from build123d import *

# Parameters (mm, degrees)
BOSS_EXTRUDE1_DEPTH = 25.4
SKETCH2_W           = 3.81
SKETCH2_H           = 30.913886478
CUT_EXTRUDE1_DEPTH  = 24.638
SKETCH3_R           = 0.1905
BOSS_EXTRUDE2_DEPTH = 27.94


with BuildPart() as part:
    # Sketch1 → Boss-Extrude1 (new body)
    with BuildSketch(Plane(origin=(0, 0, 0), x_dir=(0, 1, 0), z_dir=(0, 0, 1))):
        with BuildLine():
            Line((38.1, 31.396083107), (38.1, 54.3969813))
            Line((38.1, 54.3969813), (-38.1, 54.3969813))
            Line((-38.1, 54.3969813), (-38.1, 29.686927473))
            ThreePointArc((-38.1, 29.686927473), (-47.228063928, 16.31611269), (-50.79728762, 0.524948031))
            ThreePointArc((-50.79728762, 0.524948031), (-0.262477519, -50.799321901), (50.8, 0))
            ThreePointArc((50.8, 0), (47.722223419, 17.021685566), (38.1, 31.396083107))
        make_face()
        with BuildLine():
            Line((-38.1, 16.2969813), (-43.366277143, 9.755434728))
            ThreePointArc((-43.366277143, 9.755434728), (7.077931126, -43.882859877), (38.1, 22.895250599))
            ThreePointArc((38.1, 22.895250599), (-1.174082446, 33.154986969), (-38.1, 16.2969813))
        make_face(mode=Mode.SUBTRACT)
    extrude(amount=BOSS_EXTRUDE1_DEPTH)

    # Sketch2 → Cut-Extrude1 (cut)
    with BuildSketch(Plane.XY.offset(25.4)):
        with Locations((-52.2379813, 0.268816404)):
            Rectangle(SKETCH2_W, SKETCH2_H)
    extrude(amount=-CUT_EXTRUDE1_DEPTH, mode=Mode.SUBTRACT)

    # Sketch3 → Boss-Extrude2 (add)
    with BuildSketch(Plane.XY.offset(0.762)):
        with Locations((-52.2379813, -12.905010915)):
            Circle(SKETCH3_R)
        with Locations((-52.2379813, -9.095010915)):
            Circle(SKETCH3_R)
        with Locations((-52.2379813, -5.285010915)):
            Circle(SKETCH3_R)
        with Locations((-52.2379813, -1.475010915)):
            Circle(SKETCH3_R)
        with Locations((-52.2379813, 2.334989085)):
            Circle(SKETCH3_R)
        with Locations((-52.2379813, 6.144989085)):
            Circle(SKETCH3_R)
        with Locations((-52.2379813, 9.954989085)):
            Circle(SKETCH3_R)
        with Locations((-52.2379813, 13.764989085)):
            Circle(SKETCH3_R)
    extrude(amount=BOSS_EXTRUDE2_DEPTH)


solid = part.part
For this review, take the finished solid that the model builds, in its own axes (mm). A direction names the side the tool comes from. Round coordinates to 2 decimals unless told otherwise and drop trailing zeros. Order: outer loops, then holes, each group sorted by start corner. A loop starts at its lowest first (then second) coordinate and runs counter-clockwise, first axis right, second up. Notation, with made-up numbers: M 57.25,74 L 66.25,74 A17 cw 66.25,83 Z; hole C 41.5,84.5 d1. An arc over 180 degrees is marked long. Use a Markdown table: item, result. Add a question column.
Item 1: Tool access review of faces 1 (the cylindrical face through (-16.52, -47.14, 12.52)), 2 (the flat face through (-52, 15.726, 13)), 3 (the cylindrical face through (-33.2, -0.6, 12.5)): name each direction out of +Z, -Z, +X, -X, +Y, -Y from which nothing blocks a thin tool from reaching the whole face with its end or side.
Item 2: Add section A-A, the plane z = 16.5. State how many separate pieces and enclosed holes the cut face has, then the cut area to 3 significant figures.
Item 3: Add section D-D, the plane y = 41. Give the boundary of the cut face in (x, z).
Item 4: Insertion check: pin 1 (5 mm diameter, centred on x = 23, z = 10, fed in from -Y); pin 2 (2 mm diameter, centred on x = 30.5, y = 35, fed in from +Z); pin 3 (7.5 mm diameter, centred on x = -43, z = 9, fed in from -Y). Each pin has a flat end and moves straight along its axis. Give the tip position at first contact, or say it passes through.
Item 5: Mouldability with a two-part tool opening along Y and no side actions: class faces 4 (the flat face through (-42, -38.1, 13)), 5 (the flat face through (-54.397, 1, 13)), 6 (the flat face through (-13.07, -40.7, 12.52)), 7 (the flat face through (-43, 38.1, 13)) as released by +Y, released by -Y, zero draft, split by the parting line, or undercut.
Item 6: Add section B-B, the plane y = 0. Give the boundary of the cut face in (x, z).
Item 7: Add section C-C, the plane x = 35.5. Give the boundary of the cut face in (y, z).
Item 8: To check wall thickness, follow line 1 along X through (y, z) = (0, 7.5); line 2 along X through (y, z) = (-10, 9.5); line 3 along Y through (x, z) = (-15, 3). State the ranges of each line that lie inside material, in increasing order.
Geometry results:
| question | item | result |
|---|---|---|
| 1 | face 1 | +Z, -Z, -X, -Y |
| 1 | face 2 | +Z |
| 1 | face 3 | +Z, -Z |
| 2 | separate pieces | 9 |
| 2 | enclosed holes | 2 |
| 2 | area | 3,140 mm² |
| 3 | outline | M -28.25,0 L -17.17,0 L -17.17,25.4 L -28.25,25.4 Z; M 17.17,0 L 29.99,0 L 29.99,25.4 L 17.17,25.4 Z |
| 4 | pin 1 | stops at y = -46.48 |
| 4 | pin 2 | stops at z = 25.4 |
| 4 | pin 3 | stops at y = -38.1 |
| 5 | face 4 | released by -Y |
| 5 | face 5 | zero draft |
| 5 | face 6 | undercut |
| 5 | face 7 | released by +Y |
| 6 | outline | M -54.4,0 L -33.25,0 L -33.25,25.4 L -50.33,25.4 L -50.33,0.76 L -54.14,0.76 L -54.14,25.4 L -54.4,25.4 Z; M 44.45,0 L 50.8,0 L 50.8,25.4 L 44.45,25.4 Z |
| 7 | outline | M -36.34,0 L -26.75,0 L -26.75,25.4 L -36.34,25.4 Z; M 26.75,0 L 36.34,0 L 36.34,25.4 L 26.75,25.4 Z |
| 8 | line 1 | x = -54.4 to -54.14, -50.33 to -33.25, 44.45 to 50.8 |
| 8 | line 2 | x = -54.4 to -54.14, -50.33 to -31.73, 43.31 to 49.81 |
| 8 | line 3 | y = -47.78 to -39.14, 41.84 to 48.48 |
